Design review of the part shown in the three views and the two pictorial views. Dimensions are in mm from the part's minimum x, y and z. Coordinates: 2 decimals unless noted, no trailing zeros. Write each loop counter-clockwise with the first axis right and the second up, starting at its lowest first coordinate (ties: lowest second). Pieces come first, ordered by that corner, then holes. Notation, with made-up numbers: M 15.5,-38 L 47.5,-38 A33 ccw 47.5,-4 Z; hole C -20,-34 d2. An arc over 180 degrees is marked long. One line per question, with ' | ' between items.
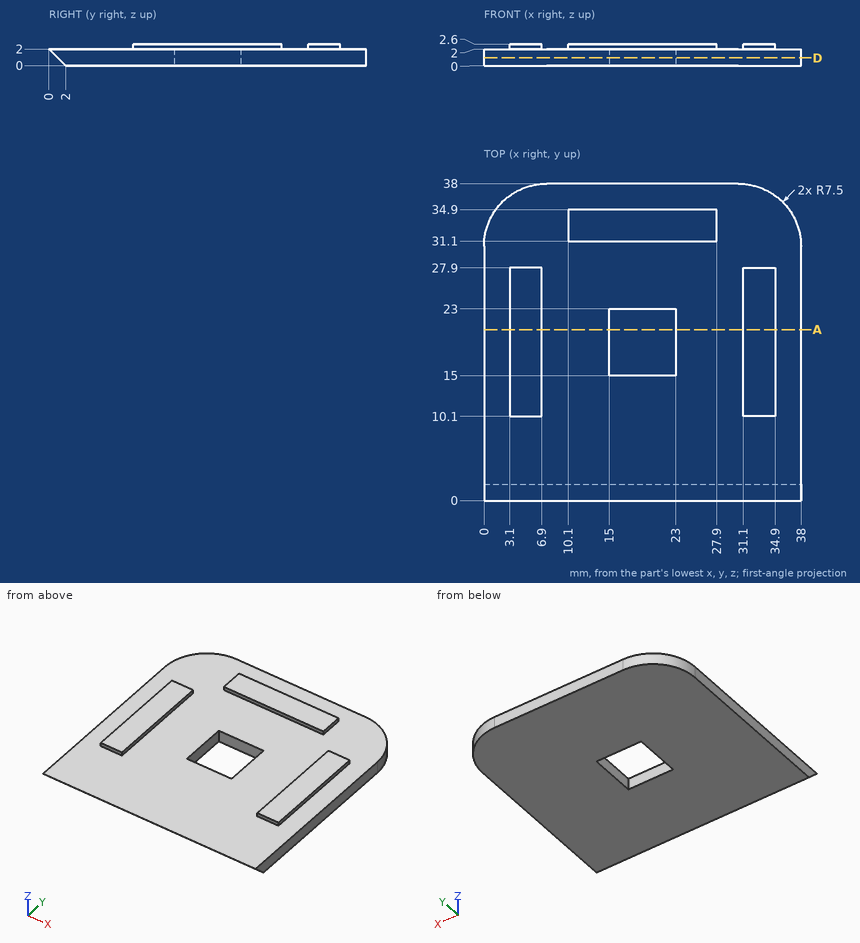
1. Take a section at A-A on y = 20.5. State the section outline as (x, z) points.
Computed values:
outline: M 0,0 L 15,0 L 15,2 L 6.9,2 L 6.9,2.6 L 3.1,2.6 L 3.1,2 L 0,2 Z; M 23,0 L 38,0 L 38,2 L 34.9,2 L 34.9,2.6 L 31.1,2.6 L 31.1,2 L 23,2 Z
2. Take a section at D-D on z = 0.95. State the section outline as (x, y) points.
Computed values:
outline: M 0,1.05 L 38,1.05 L 38,30.5 A7.5 ccw 30.5,38 L 7.5,38 A7.5 ccw 0,30.5 Z; hole M 15,15 L 23,15 L 23,23 L 15,23 Z
3. For line 1 along X through (y, z) = (17, 0.8); line 2 along X through (y, z) = (15, 2.25); line 3 along Y through (x, z) = (26, 2.45), list the stretches that pass through material, from the lowest coordinate up.
Computed values:
line 1: x = 0 to 15, 23 to 38 | line 2: x = 3.1 to 6.9, 31.1 to 34.9 | line 3: y = 31.1 to 34.9
4. Clearance check with flat-ended pins moving along their axes: P1, Ø0.5, axis at y = 17, z = 2.5, coming from the +X side; P2, Ø19, axis at x = 21.5, y = 17, coming from the +Z side; P3, Ø0.5, axis at x = 5.5, z = 2.5, coming from the -Y side. State where each tip first meets the part, or that it passes through.
Computed values:
P1: stops at x = 34.9 | P2: stops at z = 2 | P3: stops at y = 10.1
